```python
from build123d import *

# Parameters (mm, degrees)
SKETCH1_R           = 1.75
SKETCH1_W           = 55.7
SKETCH1_H           = 26
SKETCH1_W_2         = 36.5
SKETCH1_H_2         = 24
BOSS_EXTRUDE1_DEPTH = 2
SKETCH1_3_W         = 36.5
SKETCH1_3_H         = 24
SKETCH1_3_W_2       = 27.4
SKETCH1_3_H_2       = 16.5
BOSS_EXTRUDE2_DEPTH = 0.7


with BuildPart() as part:
    # Sketch1 → Boss-Extrude1 (new body)
    # profile 1 of 2: a face of its own
    with BuildSketch(Plane(origin=(0, 0, 0), x_dir=(1, 0, 0), z_dir=(0, 1, 0))):
        with BuildLine():
            Line((-39.25, 22), (28.45, 22))
            ThreePointArc((28.45, 22), (31.278427125, 20.828427125), (32.45, 18))
            Line((32.45, 18), (32.45, -18))
            ThreePointArc((32.45, -18), (31.278427125, -20.828427125), (28.45, -22))
            Line((28.45, -22), (-39.25, -22))
            ThreePointArc((-39.25, -22), (-42.078427125, -20.828427125), (-43.25, -18))
            Line((-43.25, -18), (-43.25, 18))
            ThreePointArc((-43.25, 18), (-42.078427125, 20.828427125), (-39.25, 22))
        make_face()
        with Locations(Location((-38.25, -18, 0), (0, 0, 270))):
            Circle(SKETCH1_R, mode=Mode.SUBTRACT)
        with Locations(Location((27.45, 18, 0), (0, 0, 270))):
            Circle(SKETCH1_R, mode=Mode.SUBTRACT)
        with Locations(Location((-38.25, 18, 0), (0, 0, 270))):
            Circle(SKETCH1_R, mode=Mode.SUBTRACT)
        with Locations(Location((-5.4, 18, 0), (0, 0, 270))):
            Circle(SKETCH1_R, mode=Mode.SUBTRACT)
        with Locations(Location((27.45, -18, 0), (0, 0, 270))):
            Circle(SKETCH1_R, mode=Mode.SUBTRACT)
        with Locations(Location((-5.4, -18, 0), (0, 0, 270))):
            Circle(SKETCH1_R, mode=Mode.SUBTRACT)
        with Locations((-5.4, 0)):
            Rectangle(SKETCH1_W, SKETCH1_H, mode=Mode.SUBTRACT)
    # profile 2 of 2: a face of its own
    with BuildSketch(Plane(origin=(0, 0, 0), x_dir=(1, 0, 0), z_dir=(0, 1, 0))):
        with Locations((-5.4, 0)):
            Rectangle(SKETCH1_W, SKETCH1_H)
        Rectangle(SKETCH1_W_2, SKETCH1_H_2, mode=Mode.SUBTRACT)
    extrude(amount=BOSS_EXTRUDE1_DEPTH)

    # Sketch1_3 → Boss-Extrude2 (add)
    with BuildSketch(Plane(origin=(0, 0, 0), x_dir=(1, 0, 0), z_dir=(0, 1, 0))):
        Rectangle(SKETCH1_3_W, SKETCH1_3_H)
        Rectangle(SKETCH1_3_W_2, SKETCH1_3_H_2, mode=Mode.SUBTRACT)
    extrude(amount=BOSS_EXTRUDE2_DEPTH)


solid = part.part
```
Geometry check sheet. Reference: the model listing, model coordinates, mm. A direction names the side the tool comes from. Coordinates: 2 decimals unless noted, no trailing zeros. Order: outer loops, then holes, each group sorted by start corner. A loop starts at its lowest first (then second) coordinate and runs counter-clockwise, first axis right, second up. Notation, with made-up numbers: (7.25, -13.5) - (33.25, -13.5) arc R21 ccw to (33.25, 6.5) - close; hole circle Ø7 at (78, 46.25). An arc over 180 degrees is marked (long way). Answer in a Markdown table with one row per item. Add a question column.
1. Material ranges on L1, parallel to X at y = 1.15, z = -18; L2, parallel to X at y = 1, z = 5; L3, parallel to X at y = 0.3, z = 7, recorded low to high. Write a range as [from, to].
2. Access from +Z, -Z, +X, -X, +Y, -Y to the whole of each face (thin tool, end or side, straight path). Record for faces 5 (the face through (-4.22, 0.99, -19.29)), 6 (the face through (0, 0.7, 10)).
3. Section check A-A (x = -5.4). Enter the section's corners in (y, z), plus the area to 4 significant figures.
4. Section check B-B (z = 1). Enter the section's corners in (x, y).
5. Section check C-C (y = 1.5). Enter the section's corners in (x, z).
6. Section check D-D (x = 27.45). Enter the section's corners in (y, z).
7. Gauge pin test, flat ends, axial feed: pin 1 Ø2 at (x, z) = (-38.25, 18) entering from -Y (1 decimal); pin 2 Ø1 at (x, z) = (-7, 9) entering from +Y; pin 3 Ø4.5 at (x, z) = (27.45, -18) entering from -Y. Record the tip position at first contact, or that the pin passes through.
8. Draft check along Z on faces 1 (the face through (-6, 2, -15)), 2 (the face through (-40, 1, -18)), 3 (the face through (28.63, 0.99, 16.71)), 4 (the face through (-6, 1, -22)). Enter one of: +Z half, -Z half, draft (parallel to the pull), parting line (faces both ways), or undercut.
Data:
| question | item | result |
|---|---|---|
| 1 | L1 | x = [-43.25, -40], [-36.5, -7.15], [-3.65, 25.7], [29.2, 32.45] |
| 1 | L2 | x = [-43.25, -18.25], [18.25, 32.45] |
| 1 | L3 | x = [-43.25, -13.7], [13.7, 32.45] |
| 2 | face 5 | +Y, -Y |
| 2 | face 6 | +Y |
| 3 | outline | (0, -22) - (2, -22) - (2, -19.75) - (0, -19.75) - close; (0, -16.25) - (2, -16.25) - (2, -12) - (0.7, -12) - (0.7, -8.25) - (0, -8.25) - close; (0, 8.25) - (0.7, 8.25) - (0.7, 12) - (2, 12) - (2, 16.25) - (0, 16.25) - close; (0, 19.75) - (2, 19.75) - (2, 22) - (0, 22) - close |
| 3 | area | 31.25 mm² |
| 4 | outline | (-43.25, 0) - (-13.7, 0) - (-13.7, 0.7) - (-18.25, 0.7) - (-18.25, 2) - (-43.25, 2) - close; (13.7, 0) - (32.45, 0) - (32.45, 2) - (18.25, 2) - (18.25, 0.7) - (13.7, 0.7) - close |
| 5 | outline | (-43.25, -18) arc R4 ccw to (-39.25, -22) - (28.45, -22) arc R4 ccw to (32.45, -18) - (32.45, 18) arc R4 ccw to (28.45, 22) - (-39.25, 22) arc R4 ccw to (-43.25, 18) - close; hole circle Ø3.5 at (-38.25, -18); hole circle Ø3.5 at (-38.25, 18); hole (-18.25, -12) - (18.25, -12) - (18.25, 12) - (-18.25, 12) - close; hole circle Ø3.5 at (-5.4, -18); hole circle Ø3.5 at (-5.4, 18); hole circle Ø3.5 at (27.45, -18); hole circle Ø3.5 at (27.45, 18) |
| 6 | outline | (0, -22) - (2, -22) - (2, -19.75) - (0, -19.75) - close; (0, -16.25) - (2, -16.25) - (2, 16.25) - (0, 16.25) - close; (0, 19.75) - (2, 19.75) - (2, 22) - (0, 22) - close |
| 7 | pin 1 | passes through |
| 7 | pin 2 | stops at y = 0.7 |
| 7 | pin 3 | stops at y = 0 |
| 8 | face 1 | draft |
| 8 | face 2 | undercut |
| 8 | face 3 | undercut |
| 8 | face 4 | -Z half |
